from build123d import *

# Parameters (mm, degrees)
F1_DEPTH = 19
F2_W     = 6
F2_H     = 12.5
F3_DEPTH = 571.001
F4_W     = 9.5
F4_H     = 6
F5_DEPTH = 899.001
F7_DEPTH = 19.001
F8_W     = 6
F8_H     = 6
F9_DEPTH = 571.001


with BuildPart() as f1:
    # F0 (on Right) → F1 (new body)
    with BuildSketch(Plane.YZ):
        Polygon((-496, 0), (0, 0), (0, 899), (-571, 899), (-571, 90), (-496, 90), align=None)
    extrude(amount=F1_DEPTH)

    # F2 (on Front) → F3 (cut, through all)
    with BuildSketch(Plane.XZ):
        with Locations((16, 116.25)):
            Rectangle(F2_W, F2_H)
    extrude(amount=F3_DEPTH, mode=Mode.SUBTRACT)

    # F4 (on Top) → F5 (cut, through all)
    with BuildSketch(Plane.XY):
        with Locations((14.25, -3)):
            Rectangle(F4_W, F4_H)
    extrude(amount=F5_DEPTH, mode=Mode.SUBTRACT)

    # F6 (on Right) → F7 (cut, through all)
    with BuildSketch(Plane.YZ):
        Polygon((-25, 0), (0, 0), (0, 109), (-6.915434, 90), (-25, 90), align=None)
    extrude(amount=F7_DEPTH, mode=Mode.SUBTRACT)

    # F8 (on Front) → F9 (cut, through all)
    with BuildSketch(Plane.XZ):
        with Locations((16, 896)):
            Rectangle(F8_W, F8_H)
    extrude(amount=F9_DEPTH, mode=Mode.SUBTRACT)


solid = f1.part
CAD build for the part. Positions are in the model's coordinates, mm. A direction names the side the tool comes from. Give positions to 0.01 mm unless a question says otherwise; leave off trailing zeros. Loops run counter-clockwise (first coordinate to the right, second up) from the corner with the lowest first, then second, coordinate; pieces in that order, holes last. Notation, with made-up numbers: M 67.25,79 L 115.25,79 A18 cw 115.25,110 Z; hole C 13,-9 d2. An arc over 180 degrees is marked long. Answer in a Markdown table with one row per item. Add a question column.
Item 1: Drop flat-ended pins along their axis: P1, Ø1.8, axis at y = -4, z = 308.5, coming from the +X side; P2, Ø9.5, axis at x = 5.5, y = -521.5, coming from the -Z side; P3, Ø3, axis at x = 15.5, z = 640, coming from the +Y side. Give the stop position or say it passes through.
Item 2: Band-saw the part on A-A on y = -511. Give the cut face in (x, z), then the cut area to 3 significant figures.
Item 3: Tool access for faces 1 (the face through (9, -16, 90)), 2 (the face through (19, -292, 513)), 3 (the face through (9, -534, 90)): list every direction of +Z, -Z, +X, -X, +Y, -Y with a clear straight run to the whole face (end or side of a thin tool).
Item 4: Band-saw the part on B-B on x = 6.5. Give the cut face in (y, z), then the cut area to 3 significant figures.
Item 5: Probe probe 1 along Z at (x, y) = (16.75, -67.5); probe 2 along Y at (x, z) = (11, 335); probe 3 along Z at (x, y) = (10.5, -543.5). List the from-to ranges inside material, lowest first.
Reply:
| question | item | result |
|---|---|---|
| 1 | P1 | stops at x = 9.5 |
| 1 | P2 | stops at z = 90 |
| 1 | P3 | stops at y = -6 |
| 2 | outline | M 0,90 L 19,90 L 19,110 L 13,110 L 13,122.5 L 19,122.5 L 19,893 L 13,893 L 13,899 L 0,899 Z |
| 2 | area | 15,300 mm^2 |
| 3 | face 1 | -Z, +X, -X, +Y |
| 3 | face 2 | +Z, -Z, +X, +Y, -Y |
| 3 | face 3 | -Z, +X, -X, -Y |
| 4 | outline | M -571,90 L -496,90 L -496,0 L -25,0 L -25,90 L -6.92,90 L 0,109 L 0,899 L -571,899 Z |
| 4 | area | 504,000 mm^2 |
| 5 | probe 1 | z = 0 to 110, 122.5 to 893 |
| 5 | probe 2 | y = -571 to -6 |
| 5 | probe 3 | z = 90 to 899 |
